Can you work these out from the model? Positions are in its coordinate system, mm. Round coordinates to 2 decimals unless told otherwise and drop trailing zeros. Loops run counter-clockwise (first coordinate to the right, second up) from the corner with the lowest first, then second, coordinate; pieces in that order, holes last.
from build123d import *

# Parameters (mm, degrees)
F0_W     = 100
F0_H     = 50
F1_DEPTH = 10
F3_D     = 6.8
F4_SIZE  = 5


with BuildPart() as f1:
    # F0 (on Top) → F1 (new body, symmetric)
    with BuildSketch(Plane.XY):
        Rectangle(F0_W, F0_H)
    extrude(amount=F1_DEPTH, both=True)

    # F3 (through all)
    with Locations(Plane.XY.offset(10)):
        with Locations((0, 0)):
            Hole(F3_D / 2)

    # F4
    f4_edges = [f1.edges().sort_by_distance(p)[0] for p in [
        (-50, 0, 10),
        (0, -25, 10),
        (50, 0, 10),
        (0, 25, 10),
    ]]
    chamfer(f4_edges, length=F4_SIZE)


solid = f1.part
(1) If we mould it in two halves opening along Y, with no side actions, what happens to faces 1 (the flat face through (-1, 6, -10)), 2 (the cylindrical face through (0.74, -3.32, -0.14)), 3 (the flat face through (-1, 22, 8))? For each: released by +Y, released by -Y, zero draft, split by the parting line, or undercut.
Worked answers:
face 1: zero draft
face 2: undercut
face 3: released by +Y
(2) If I drill on line 1 (Y direction, x = 0, z = 2.5); line 2 (X direction, y = 2.5, z = -6.75); line 3 (Z direction, x = -41, y = -22), over which ranges is the centre line in solid material (lowest first)?
Worked answers:
line 1: y = -25 to -3.4, 3.4 to 25
line 2: x = -50 to -2.3, 2.3 to 50
line 3: z = -10 to 8
(3) Will this pin go through, and if not, where does the flat tip stop? P1, Ø1, axis at x = 8, z = 6, coming from the +Y side.
Worked answers:
P1: stops at y = 24.5
(4) If we section it at B-B, the plane x = 0: List the corners of the cut face in (y, z) for me.
Worked answers:
outline: (-25, -10) - (-3.4, -10) - (-3.4, 10) - (-20, 10) - (-25, 5) - close; (3.4, -10) - (25, -10) - (25, 5) - (20, 10) - (3.4, 10) - close
(5) If we section it at C-C, the plane z = 6.75: List the corners of the cut face in (x, y) for me, then the cut area to 3 significant figures.
Worked answers:
outline: (-48.25, -23.25) - (48.25, -23.25) - (48.25, 23.25) - (-48.25, 23.25) - close; hole circle Ø6.8 at (0, 0)
area: 4,450 mm2
(6) If we section it at D-D, the plane y = -21: List the corners of the cut face in (x, z) for me.
Worked answers:
outline: (-50, -10) - (50, -10) - (50, 5) - (46, 9) - (-46, 9) - (-50, 5) - close
(7) If we section it at A-A, the plane y = 0: List the corners of the cut face in (x, z) for me, then the cut area to 3 significant figures.
Worked answers:
outline: (-50, -10) - (-3.4, -10) - (-3.4, 10) - (-45, 10) - (-50, 5) - close; (3.4, -10) - (50, -10) - (50, 5) - (45, 10) - (3.4, 10) - close
area: 1,840 mm2
